The model under review builds one solid part; all positions refer to its coordinate system, in mm. Give positions to 0.01 mm unless a question says otherwise; leave off trailing zeros. Order: outer loops, then holes, each group sorted by start corner. A loop starts at its lowest first (then second) coordinate and runs counter-clockwise, first axis right, second up. Notation, with made-up numbers: (11.25, 81.25) -> (68.25, 81.25) arc R17 ccw to (68.25, 107.25) -> close; hole circle Ø8 at (-36.5, 71). An arc over 180 degrees is marked (long way). Use one line per item in the form item = value.
```python
from build123d import *

# Parameters (mm, degrees)
SKETCH_2_W        = 10
SKETCH_2_H        = 10
EXTRUDE_1_DEPTH   = 30
EXTRUDE_1_2_DEPTH = 30
EXTRUDE_1_3_DEPTH = 30
EXTRUDE_1_4_DEPTH = 30
SKETCH_3_W        = 284.641016152
SKETCH_3_H        = 100
EXTRUDE_2_DEPTH   = 3
SKETCH_4_W        = 244.638026471
SKETCH_4_H        = 5
EXTRUDE_3_DEPTH   = 23


with BuildPart() as part:
    # Sketch 2 → Extrude 1 (new body)
    with BuildSketch(Plane(origin=(0, 0, 0), x_dir=(1, 0, 0), z_dir=(0, 1, 0))):
        with Locations((-132.320508076, 40)):
            Rectangle(SKETCH_2_W, SKETCH_2_H)
    extrude(amount=EXTRUDE_1_DEPTH)



with BuildPart() as body_2:
    # Sketch 2 → Extrude 1 2 (new body)
    with BuildSketch(Plane(origin=(0, 0, 0), x_dir=(1, 0, 0), z_dir=(0, 1, 0))):
        with Locations((-132.320508076, -40)):
            Rectangle(SKETCH_2_W, SKETCH_2_H)
    extrude(amount=EXTRUDE_1_2_DEPTH)


with BuildPart() as body_3:
    # Sketch 2 → Extrude 1 3 (new body)
    with BuildSketch(Plane(origin=(0, 0, 0), x_dir=(1, 0, 0), z_dir=(0, 1, 0))):
        with Locations((132.320508076, -40)):
            Rectangle(SKETCH_2_W, SKETCH_2_H)
    extrude(amount=EXTRUDE_1_3_DEPTH)


with BuildPart() as body_4:
    # Sketch 2 → Extrude 1 4 (new body)
    with BuildSketch(Plane(origin=(0, 0, 0), x_dir=(1, 0, 0), z_dir=(0, 1, 0))):
        with Locations((132.320508076, 40)):
            Rectangle(SKETCH_2_W, SKETCH_2_H)
    extrude(amount=EXTRUDE_1_4_DEPTH)


with BuildPart() as part_1:
    add(part.part)

    add(body_2.part)  # Extrude 2 merges body 2

    add(body_3.part)  # Extrude 2 merges body 3

    add(body_4.part)  # Extrude 2 merges body 4
    # Sketch 3 → Extrude 2 (add)
    with BuildSketch(Plane(origin=(0, 0, 0), x_dir=(1, 0, 0), z_dir=(0, 1, 0))):
        Rectangle(SKETCH_3_W, SKETCH_3_H)
    extrude(amount=-EXTRUDE_2_DEPTH)

    # Sketch 4 → Extrude 3 (add)
    with BuildSketch(Plane(origin=(0, 0, 0), x_dir=(1, 0, 0), z_dir=(0, 1, 0))):
        with Locations((-0.001494841, 47.5)):
            Rectangle(SKETCH_4_W, SKETCH_4_H)
    extrude(amount=EXTRUDE_3_DEPTH)


solid = part_1.part
```
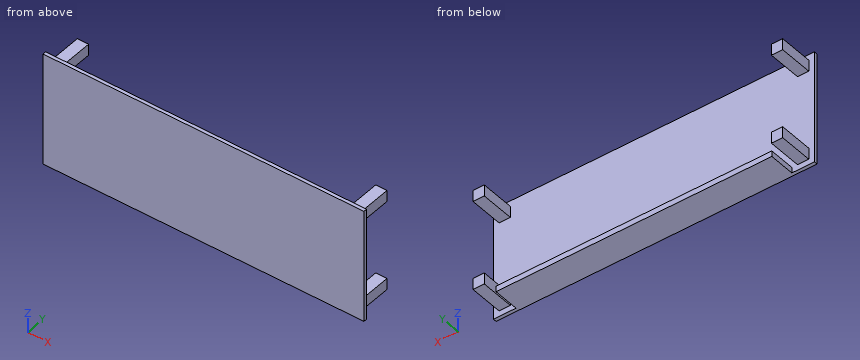
1. For pin 1 Ø5 at (x, y) = (-133.5, 9.5) entering from +Z; pin 2 Ø6 at (y, z) = (5, 9.5) entering from -X; pin 3 Ø3 at (x, y) = (-130, 11.5) entering from -Z; pin 4 Ø6 at (y, z) = (12, 39) entering from +X, all flat-tipped, find the tip position at first contact; note any pin that passes through.
Values:
pin_1 = 45
pin_2 = through
pin_3 = -45
pin_4 = 137.32
2. Add section C-C on z = 29. Give the boundary of the cut face in (x, y).
Values:
outline = (-142.32, -3) -> (142.32, -3) -> (142.32, 0) -> (-142.32, 0) -> close
3. Add section B-B on x = -45. Give the boundary of the cut face in (y, z).
Values:
outline = (-3, -50) -> (23, -50) -> (23, -45) -> (0, -45) -> (0, 50) -> (-3, 50) -> close
4. For L1, parallel to X at y = 3.5, z = 40; L2, parallel to Y at x = -59, z = -37.5; L3, parallel to Z at x = -117, y = 3, list the stretches that pass through material, from the lowest coordinate up.
Values:
L1 = -137.32 to -127.32, 127.32 to 137.32
L2 = -3 to 0
L3 = -50 to -45
5. Add section A-A on y = 5.5. Give the boundary of the cut face in (x, z), then the cut area to 3 significant figures.
Values:
outline = (-137.32, -45) -> (-127.32, -45) -> (-127.32, -35) -> (-137.32, -35) -> close; (-137.32, 35) -> (-127.32, 35) -> (-127.32, 45) -> (-137.32, 45) -> close; (-122.32, -50) -> (122.32, -50) -> (122.32, -45) -> (-122.32, -45) -> close; (127.32, -45) -> (137.32, -45) -> (137.32, -35) -> (127.32, -35) -> close; (127.32, 35) -> (137.32, 35) -> (137.32, 45) -> (127.32, 45) -> close
area = 1,620 mm^2
